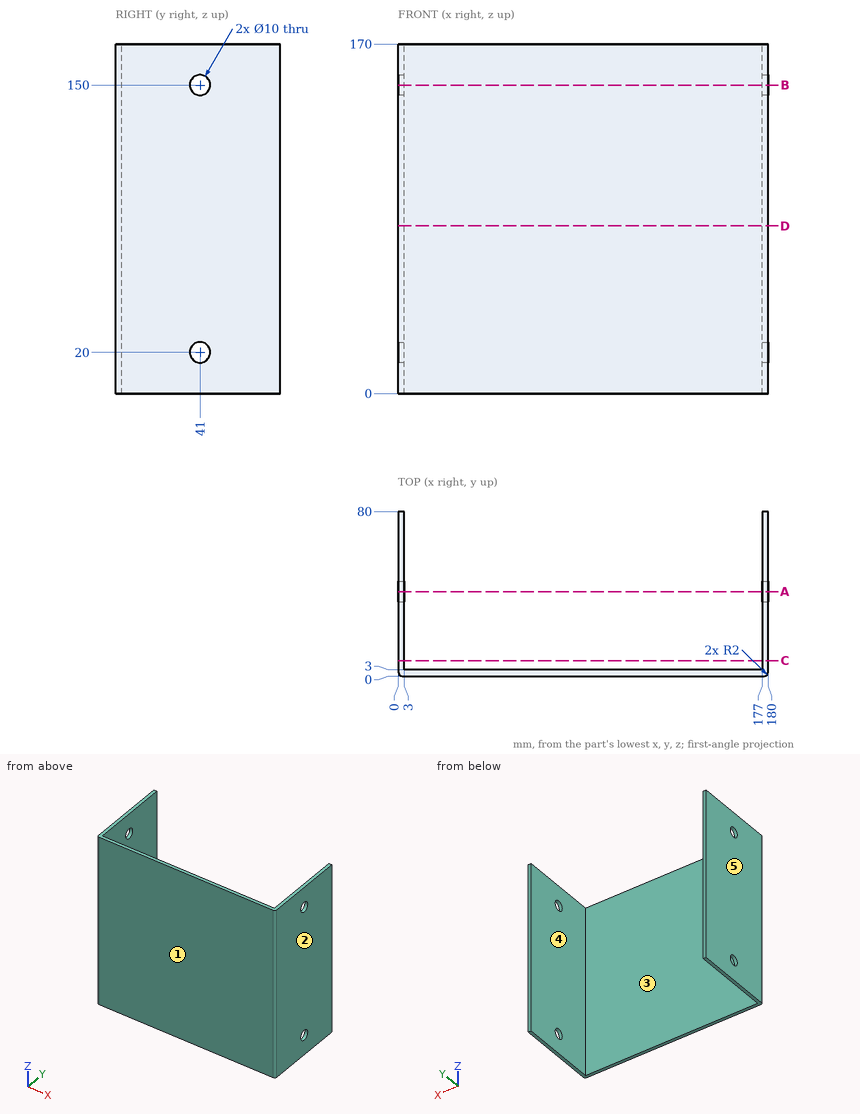
Study the drawing (mm; zero at the part's minimum x, y, z) and answer. A direction names the side the tool comes from. Coordinates: 2 decimals unless noted, no trailing zeros. Loops run counter-clockwise (first coordinate to the right, second up) from the corner with the lowest first, then second, coordinate; pieces in that order, holes last. Notation, with made-up numbers: (36.25, 13) -> (72.25, 13) arc R16 cw to (72.25, 37) -> close; hole circle Ø1 at (-16, 8.5). An arc over 180 degrees is marked (long way). Write each question's results on one line, items separated by ' | '. Start each with the question number.
1) For the marked faces 4 and 5, determine the directions among +Z, -Z, +X, -X, +Y, -Y from which every point of the face is accessible in a straight line to the end or side of a thin tool.
2) Find section B-B on z = 150. Determine the outline of the cut face in (x, y), then the cut area to 3 significant figures.
3) Find section D-D on z = 81.5. Determine the outline of the cut face in (x, y), then the cut area to 3 significant figures.
4) Consider line 1 along Y through (x, z) = (2.3, 150); line 2 along X through (y, z) = (17, 129); line 3 along Y through (x, z) = (98, 104). Determine where each line is inside the solid, lowest interval first.
5) Find section A-A on y = 41. Determine the outline of the cut face in (x, z).
6) Flat-ended cylindrical pins translate along their axes: P1, Ø11.5, axis at y = 41, z = 150, coming from the -X side; P2, Ø1.5, axis at x = 59, z = 150, coming from the +Y side. Find the tip coordinate at first contact, or state that the pin passes through.
7) Find section C-C on y = 7.5. Determine the outline of the cut face in (x, z), then the cut area to 3 significant figures.
8) The mould has two halves that part along X. Classify the marked faces 1, 2 and 3: pulls with the +X half, pulls with the -X half, needs draft (parallel to the pull), parting line crosses it, or undercut.
Response values:
1) face 4: +Z, -Z, +Y | face 5: +Z, -Z, -X, +Y, -Y
2) outline: (0, 2) arc R2 ccw to (2, 0) -> (178, 0) arc R2 ccw to (180, 2) -> (180, 36) -> (177, 36) -> (177, 3) -> (3, 3) -> (3, 36) -> (0, 36) -> close; (0, 46) -> (3, 46) -> (3, 80) -> (0, 80) -> close; (177, 46) -> (180, 46) -> (180, 80) -> (177, 80) -> close | area: 940 mm^2
3) outline: (0, 2) arc R2 ccw to (2, 0) -> (178, 0) arc R2 ccw to (180, 2) -> (180, 80) -> (177, 80) -> (177, 3) -> (3, 3) -> (3, 80) -> (0, 80) -> close | area: 1,000 mm^2
4) line 1: y = 0 to 36, 46 to 80 | line 2: x = 0 to 3, 177 to 180 | line 3: y = 0 to 3
5) outline: (0, 0) -> (3, 0) -> (3, 15) -> (0, 15) -> close; (0, 25) -> (3, 25) -> (3, 145) -> (0, 145) -> close; (0, 155) -> (3, 155) -> (3, 170) -> (0, 170) -> close; (177, 0) -> (180, 0) -> (180, 15) -> (177, 15) -> close; (177, 25) -> (180, 25) -> (180, 145) -> (177, 145) -> close; (177, 155) -> (180, 155) -> (180, 170) -> (177, 170) -> close
6) P1: stops at x = 0 | P2: stops at y = 3
7) outline: (0, 0) -> (3, 0) -> (3, 170) -> (0, 170) -> close; (177, 0) -> (180, 0) -> (180, 170) -> (177, 170) -> close | area: 1,020 mm^2
8) face 1: needs draft | face 2: pulls with the +X half | face 3: undercut
